Source: CAD feature listing. Evaluate the final solid. Frame: model axes, mm. Face numbers are marked on the shaded views. Round coordinates to 2 decimals unless told otherwise and drop trailing zeros. Write each loop counter-clockwise with the first axis right and the second up, starting at its lowest first coordinate (ties: lowest second). Pieces come first, ordered by that corner, then holes. Notation, with made-up numbers: M -23,40.25 L -7,40.25 A35 cw -7,78.25 Z; hole C 77,48.5 d1. An arc over 180 degrees is marked long. Use a Markdown table: item, result.
```python
from build123d import *

# Parameters (mm, degrees)
SKETCH1_W           = 50
SKETCH1_H           = 50
SKETCH1_R           = 7.5
BOSS_EXTRUDE1_DEPTH = 10


with BuildPart() as part:
    # Sketch1 → Boss-Extrude1 (new, symmetric)
    with BuildSketch(Plane(origin=(0, 0, 0), x_dir=(1, 0, 0), z_dir=(0, 1, 0))):
        Rectangle(SKETCH1_W, SKETCH1_H)
        with Locations(Location((0, 0, 0), (0, 0, 270))):
            Circle(SKETCH1_R, mode=Mode.SUBTRACT)
    extrude(amount=BOSS_EXTRUDE1_DEPTH, both=True)


solid = part.part
```
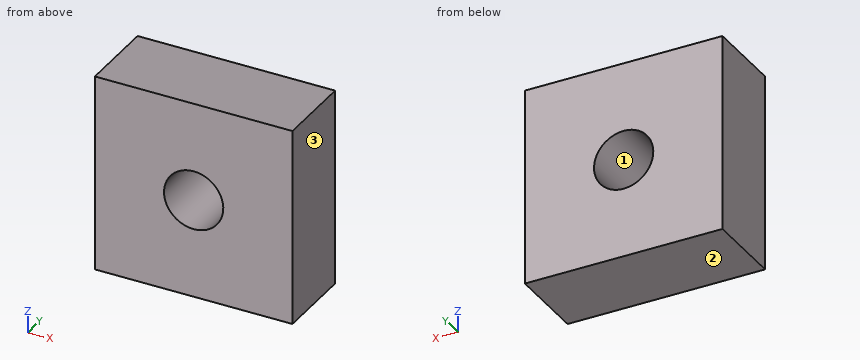
Q1. Line query: L1, parallel to X at y = -4.25, z = 0; L2, parallel to Z at x = -4, y = 6.5; L3, parallel to X at y = -5.25, z = 2. Output: solid intervals per line, ascending.
Results are:
| item | result |
|---|---|
| L1 | -25 to -7.5, 7.5 to 25 |
| L2 | -25 to -6.34, 6.34 to 25 |
| L3 | -25 to -7.23, 7.23 to 25 |
Q2. Section B-B on x = 0. Return loops of the section in (y, z), plus the area to 3 significant figures.
Results are:
| item | result |
|---|---|
| outline | M -10,-25 L 10,-25 L 10,-7.5 L -10,-7.5 Z; M -10,7.5 L 10,7.5 L 10,25 L -10,25 Z |
| area | 700 mm^2 |
Q3. Mould query, pull axis X, two halves, no side actions, for the marked faces 1, 2 and 3. Classes: +X half, -X half, draft (parallel to the pull), parting line (faces both ways), or undercut.
Results are:
| item | result |
|---|---|
| face 1 | undercut |
| face 2 | draft |
| face 3 | +X half |
Q4. Section C-C on y = -3.5. Return loops of the section in (x, z), plus the area to 3 significant figures.
Results are:
| item | result |
|---|---|
| outline | M -25,-25 L 25,-25 L 25,25 L -25,25 Z; hole C 0,0 d15 |
| area | 2,320 mm^2 |
Q5. Section A-A on z = 0. Return loops of the section in (x, y).
Results are:
| item | result |
|---|---|
| outline | M -25,-10 L -7.5,-10 L -7.5,10 L -25,10 Z; M 7.5,-10 L 25,-10 L 25,10 L 7.5,10 Z |
